from build123d import *

# Parameters (mm, degrees)
F0_R     = 6.35
F1_DEPTH = 63.5
F2_R     = 2.2225
F3_DEPTH = 3.175
F5_DEPTH = 12.7


with BuildPart() as f1:
    # F0 (on Top) → F1 (new body)
    with BuildSketch(Plane.XY):
        Circle(F0_R)
    extrude(amount=F1_DEPTH)

    # F2 (on face) → F3 (join)
    with BuildSketch(Plane.XY.offset(63.5)):
        Circle(F2_R)
    extrude(amount=F3_DEPTH)

    # F4 (on face) → F5 (join)
    with BuildSketch(Plane.XY.offset(66.675)):
        with BuildLine():
            ThreePointArc((-2.182627, -0.4191), (0, -2.2225), (2.182627, -0.4191))
            Line((2.182627, -0.4191), (-2.182627, -0.4191))
        make_face()
        with BuildLine():
            ThreePointArc((2.182627, 0.4191), (0, 2.2225), (-2.182627, 0.4191))
            Line((-2.182627, 0.4191), (2.182627, 0.4191))
        make_face()
    extrude(amount=F5_DEPTH)


solid = f1.part
Work out the finished part from the listing and answer in its coordinate system (mm). A direction names the side the tool comes from. Give positions to 0.01 mm unless a question says otherwise; leave off trailing zeros. Order: outer loops, then holes, each group sorted by start corner. A loop starts at its lowest first (then second) coordinate and runs counter-clockwise, first axis right, second up. Notation, with made-up numbers: (38.25, 38.5) -> (82.25, 38.5) arc R34 cw to (82.25, 77.5) -> close; hole circle Ø7 at (-1.5, 24.5). An arc over 180 degrees is marked (long way). Answer as a JSON object with one key per item and string values. Group by question number.
1. Consider line 1 along Z through (x, y) = (1, 4.25); line 2 along Y through (x, z) = (3.25, 53); line 3 along X through (y, z) = (4, 4.5). Determine where each line is inside the solid, lowest interval first. Write a range as [from, to].
2. Section B-B on y = -1.5 is taken. Determine the outline of the cut face in (x, z) (3 decimals), plus the area to 3 significant figures.
3. Section D-D on x = -4.5 is taken. Determine the outline of the cut face in (y, z).
4. The mould has two halves that part along Y. Classify faces 4 (the flat face through (0, -1, 79.375)), 5 (the cylindrical face through (-1.38, -6.2, 31.31)), 6 (the flat face through (0, -0.419, 73)): released by +Y, released by -Y, zero draft, split by the parting line, or undercut.
5. Section C-C on z = 9 is taken. Determine the outline of the cut face in (x, y), plus the area to 3 significant figures.
6. Flat-ended cylindrical pins translate along their axes: pin 1 Ø1 at (x, z) = (-1, 65) entering from +Y; pin 2 Ø1.5 at (x, y) = (3.5, -3.5) entering from +Z; pin 3 Ø3 at (x, z) = (3.5, 47) entering from -Y. Find the tip coordinate at first contact, or state that the pin passes through.
7. A tool of negligible diameter and unlimited length cuts with its end or side. For faces 1 (the flat face through (0, 0, 0)), 2 (the flat face through (0, 0.419, 73)), 3 (the flat face through (3, 0, 63.5)), from which of +Z, -Z, +X, -X, +Y, -Y can it reach the whole face along a straight path? Write none if from no direction.
Result sheet:
{
 "1": {"line 1": "z = [0, 63.5]", "line 2": "y = [-5.46, 5.46]", "line 3": "x = [-4.93, 4.93]"},
 "2": {"outline": "(-6.17, 0) -> (6.17, 0) -> (6.17, 63.5) -> (1.64, 63.5) -> (1.64, 79.375) -> (-1.64, 79.375) -> (-1.64, 63.5) -> (-6.17, 63.5) -> close", "area": "836 mm^2"},
 "3": {"outline": "(-4.48, 0) -> (4.48, 0) -> (4.48, 63.5) -> (-4.48, 63.5) -> close"},
 "4": {"face 4": "zero draft", "face 5": "split by the parting line", "face 6": "undercut"},
 "5": {"outline": "circle Ø12.7 at (0, 0)", "area": "127 mm^2"},
 "6": {"pin 1": "stops at y = 2.17", "pin 2": "stops at z = 63.5", "pin 3": "stops at y = -6.03"},
 "7": {"face 1": "-Z, +X, -X, +Y, -Y", "face 2": "+Z, +X, -X", "face 3": "+Z"}
}
